CAD build for the part. Positions are in the model's coordinates, mm. Face numbers are marked on the shaded views. A direction names the side the tool comes from. Coordinates: 2 decimals unless noted, no trailing zeros. Write each loop counter-clockwise with the first axis right and the second up, starting at its lowest first coordinate (ties: lowest second). Pieces come first, ordered by that corner, then holes. Notation, with made-up numbers: (37, 17.25) - (44, 17.25) arc R19 cw to (44, 41.25) - close; hole circle Ø11 at (-20, -5). An arc over 180 degrees is marked (long way). Answer in a Markdown table with one row per item. Add a question column.
Q1. 3-axis set-ups, long thin cutter, end or side, ignore diameter. For the marked faces 4, 5 and 6: which of +Z, -Z, +X, -X, +Y, -Y reach the whole face in a straight line?
Q2. Two-plate mould, pull along Z, no slides. Class the marked faces 1, 2 and 3: +Z half, -Z half, draft (parallel to the pull), parting line (faces both ways), or undercut.
Q3. Pin check, flat tip, straight feed: pin 1 (10 mm diameter, centred on y = -87.5, z = -13, fed in from +X). Stop position of the tip, or through.
Q4. Band-saw the part on B-B (z = -93). List the corners of the cut face in (x, y), and give its area (3 significant figures).
Q5. Band-saw the part on A-A (z = -54.5). List the corners of the cut face in (x, y).
Q6. Band-saw the part on C-C (x = -67). List the corners of the cut face in (y, z).
Q7. Drill centre lines: line 1 along Z through (x, y) = (-69, -113.5); line 2 along Y through (x, z) = (-68.5, -16); line 3 along X through (y, z) = (-102, -59.5). Where is each one in solid material? Low to high. Write a range as from..to.
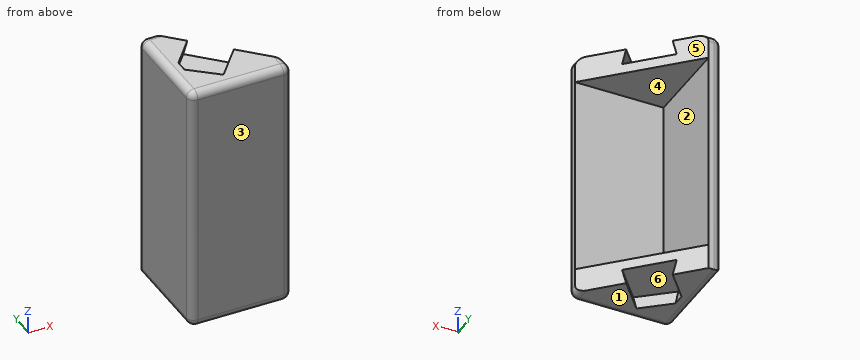
```python
from build123d import *

# Parameters (mm, degrees)
EXTRUDE_1_DEPTH = 10
EXTRUDE_3_DEPTH = 40
FILLET_2_R      = 3
FILLET_3_R      = 3


with BuildPart() as part:
    # 草图3 → 凸台-拉伸1 (new body)
    with BuildSketch(Plane.XY):
        Polygon((-100, -79.175359259), (-100, -119.175359259), (-60, -119.175359259), (-60, -114.175359259), (-95, -79.175359259), align=None)
    extrude(amount=-EXTRUDE_1_DEPTH)

    # 草图5 → 切除-放样1 section 0
    with BuildSketch(Plane.XY.offset(-6)):
        with BuildLine():
            Line((-96.08, -104.799041882), (-96.08, -98.821989002))
            Line((-96.08, -98.821989002), (-81.709132385, -81.695455893))
            Line((-81.709132385, -81.695455893), (-66.265676412, -94.654054104))
            Line((-66.265676412, -94.654054104), (-83.579668035, -115.288065824))
            Line((-83.579668035, -115.288065824), (-96.08, -104.799041882))
        make_face()
    # 草图8 → 切除-放样1 section 1
    with BuildSketch(Plane.XY):
        with BuildLine():
            Line((-94.58, -104.099580395), (-94.58, -99.367944353))
            Line((-94.58, -99.367944353), (-80.56006572, -82.659637307))
            Line((-80.56006572, -82.659637307), (-67.414743077, -93.68987269))
            Line((-67.414743077, -93.68987269), (-83.764553285, -113.174817744))
            Line((-83.764553285, -113.174817744), (-94.58, -104.099580395))
        make_face()
    loft(mode=Mode.SUBTRACT)

    # 草图9 → 凸台-拉伸3 (add)
    with BuildSketch(Plane(origin=(0, 0, -10), x_dir=(-1, 0, 0), z_dir=(0, 0, -1))):
        Polygon((95, -79.175359259), (95, -114.175359259), (60, -114.175359259), (60, -119.175359259), (100, -119.175359259), (100, -79.175359259), align=None)
    extrude(amount=EXTRUDE_3_DEPTH)

    # 镜向2: part across plane


with BuildPart() as part_1:
    add(part.part)
    add(part.part.mirror(Plane(origin=(0, 0, -50), x_dir=(1, 0, 0), z_dir=(0, 0, -1))))

    # 圆角2
    fillet_2_edges = [part_1.edges().sort_by_distance(p)[0] for p in [
        (-60, -116.675359259, -100),
        (-60, -116.675359259, 0),
        (-100, -99.175359259, -100),
        (-100, -99.175359259, 0),
        (-100, -79.175359259, -50),
        (-97.5, -79.175359259, 0),
    ]]
    fillet(fillet_2_edges, radius=FILLET_2_R)

    # 圆角3
    fillet_3_edges = [part_1.edges().sort_by_distance(p)[0] for p in [
        (-80, -119.175359259, -100),
        (-80, -119.175359259, 0),
        (-100, -119.175359259, -50),
        (-60, -119.175359259, -50),
        (-99.121320344, -119.175359259, -0.878679656),
        (-99.121320344, -119.175359259, -99.121320344),
        (-60.878679656, -119.175359259, -0.878679656),
        (-60.878679656, -119.175359259, -99.121320344),
    ]]
    fillet(fillet_3_edges, radius=FILLET_3_R)


solid = part_1.part
```
Checked values:
| question | item | result |
|---|---|---|
| 1 | face 4 | +X, +Y |
| 1 | face 5 | +Z, -Z, +X, +Y |
| 1 | face 6 | none |
| 2 | face 1 | -Z half |
| 2 | face 2 | undercut |
| 2 | face 3 | draft |
| 3 | pin 1 | stops at x = -82.68 |
| 4 | outline | (-100, -116.18) arc R3 ccw to (-97, -119.18) - (-63, -119.18) arc R3 ccw to (-60, -116.18) - (-60, -114.18) - (-95, -79.18) - (-97, -79.18) arc R3 ccw to (-100, -82.18) - close |
| 4 | area | 982 mm² |
| 5 | outline | (-100, -116.18) arc R3 ccw to (-97, -119.18) - (-63, -119.18) arc R3 ccw to (-60, -116.18) - (-60, -114.18) - (-95, -114.18) - (-95, -79.18) - (-97, -79.18) arc R3 ccw to (-100, -82.18) - close |
| 6 | outline | (-119.18, -97) arc R3 ccw to (-116.18, -100) - (-107.18, -100) - (-107.18, -90) - (-114.18, -90) - (-114.18, -10) - (-107.18, -10) - (-107.18, 0) - (-116.18, 0) arc R3 ccw to (-119.18, -3) - close |
| 7 | line 1 | z = -100..-90, -10..0 |
| 7 | line 2 | y = -119.18..-114.18 |
| 7 | line 3 | x = -100..-95 |
